The model under review builds one solid part; all positions refer to its coordinate system, in mm. A direction names the side the tool comes from. Round coordinates to 2 decimals unless told otherwise and drop trailing zeros. Loops run counter-clockwise (first coordinate to the right, second up) from the corner with the lowest first, then second, coordinate; pieces in that order, holes last. Notation, with made-up numbers: (36, -7) -> (69, -7) arc R28 cw to (69, 11) -> close; hole circle Ø4 at (-24.75, 88). An arc over 180 degrees is marked (long way). Use CSV: the item, a comma, the result in double quotes. Start each with the question number.
```python
from build123d import *

# Parameters (mm, degrees)
F0_R     = 7.366
F0_R_2   = 5.7785
F1_DEPTH = 1
F2_DEPTH = 2.032
F4_DEPTH = 7.366


with BuildPart() as f1:
    # F0 (on Top) → F1 (new body)
    with BuildSketch(Plane.XY):
        Circle(F0_R)
        Circle(F0_R_2, mode=Mode.SUBTRACT)
        Circle(F0_R_2)
    extrude(amount=F1_DEPTH)

    # F0 (on Top) → F2 (join)
    with BuildSketch(Plane.XY):
        Circle(F0_R)
        Circle(F0_R_2, mode=Mode.SUBTRACT)
    extrude(amount=F2_DEPTH)

    # F3 (on face) → F4 (join)
    with BuildSketch(Plane.XY.offset(1)):
        with BuildLine():
            ThreePointArc((-3.1130078892, 3.687744281), (0, 4.826), (3.1130078892, 3.687744281))
            Line((3.1130078892, 3.687744281), (3.7885305572, 4.3632669489))
            ThreePointArc((3.7885305572, 4.3632669489), (0, 5.7785), (-3.7885305572, 4.3632669489))
            Line((-3.7885305572, 4.3632669489), (-3.1130078892, 3.687744281))
        make_face()
        with BuildLine():
            ThreePointArc((-3.687744281, -3.1130078892), (-4.826, 0), (-3.687744281, 3.1130078892))
            Line((-3.687744281, 3.1130078892), (-4.3632669489, 3.7885305572))
            ThreePointArc((-4.3632669489, 3.7885305572), (-5.7785, 0), (-4.3632669489, -3.7885305572))
            Line((-4.3632669489, -3.7885305572), (-3.687744281, -3.1130078892))
        make_face()
        with BuildLine():
            Line((3.7885305572, -4.3632669489), (3.1130078892, -3.687744281))
            ThreePointArc((3.1130078892, -3.687744281), (0, -4.826), (-3.1130078892, -3.687744281))
            Line((-3.1130078892, -3.687744281), (-3.7885305572, -4.3632669489))
            ThreePointArc((-3.7885305572, -4.3632669489), (0, -5.7785), (3.7885305572, -4.3632669489))
        make_face()
        with BuildLine():
            ThreePointArc((3.687744281, 3.1130078892), (4.5325119912, 1.6572902733), (4.826, 0))
            ThreePointArc((4.826, 0), (4.5325119912, -1.6572902733), (3.687744281, -3.1130078892))
            Line((3.687744281, -3.1130078892), (4.3632669489, -3.7885305572))
            ThreePointArc((4.3632669489, -3.7885305572), (5.4131414315, -2.0221182193), (5.7785, 0))
            ThreePointArc((5.7785, 0), (5.4131414315, 2.0221182193), (4.3632669489, 3.7885305572))
            Line((4.3632669489, 3.7885305572), (3.687744281, 3.1130078892))
        make_face()
    extrude(amount=F4_DEPTH)


solid = f1.part
```
1. For line 1 along Z through (x, y) = (2.75, -0.5); line 2 along Y through (x, z) = (-0.25, 3.75); line 3 along Y through (x, z) = (-2.5, 3.5), list the stretches that pass through material, from the lowest coordinate up. Write a range as from..to.
2. Take a section at C-C, the plane x = 0. Give the boundary of the cut face in (y, z).
3. Take a section at B-B, the plane z = 1.75. Give the boundary of the cut face in (x, y), then the cut area to 3 significant figures.
4. For faces 1 (the face through (0, 0, 1)), 2 (the face through (-5.78, 0.06, 5.15)), 3 (the face through (0.06, 5.78, 5.15)), list the 3-axis set-ups (+Z, -Z, +X, -X, +Y, -Y) from which the entire face can be reached by the end or side of a thin tool; tool diameter is ignored.
5. Clearance check with a flat-ended pin moving along its axis: P1, Ø2, axis at y = -2, z = 2, coming from the +X side. State where the tip first meets the part, or that it passes through.
6. Take a section at A-A, the plane z = 7. Give the boundary of the cut face in (x, y), then the cut area to 3 significant figures.
7. The part is to be moulded in two halves that separate along X. For faces 4 (the face through (0.047, -4.826, 4.631)), 5 (the face through (-4.826, -0.047, 4.631)), 6 (the face through (5, 0, 8.366)), 7 (the face through (-0.06, -5.78, 5.15)), say which applies: pulls with the +X half, pulls with the -X half, needs draft (parallel to the pull), parting line crosses it, or undercut.
8. Take a section at D-D, the plane y = -1.5. Give the boundary of the cut face in (x, z).
Results:
1,line 1,"0..1"
1,line 2,"-5.77..-4.82, 4.82..5.77"
1,line 3,"-5.21..-4.13, 4.13..5.21"
2,outline,"(-7.37, 0) -> (7.37, 0) -> (7.37, 2.03) -> (5.78, 2.03) -> (5.78, 8.37) -> (4.83, 8.37) -> (4.83, 1) -> (-4.83, 1) -> (-4.83, 8.37) -> (-5.78, 8.37) -> (-5.78, 2.03) -> (-7.37, 2.03) -> close"
3,outline,"circle Ø14.73 at (0, 0); hole (-4.36, -3.79) arc R5.78 ccw to (-3.79, -4.36) -> (-3.11, -3.69) arc R4.83 ccw to (3.11, -3.69) -> (3.79, -4.36) arc R5.78 ccw to (4.36, -3.79) -> (3.69, -3.11) arc R4.83 ccw to (3.69, 3.11) -> (4.36, 3.79) arc R5.78 ccw to (3.79, 4.36) -> (3.11, 3.69) arc R4.83 ccw to (-3.11, 3.69) -> (-3.79, 4.36) arc R5.78 ccw to (-4.36, 3.79) -> (-3.69, 3.11) arc R4.83 ccw to (-3.69, -3.11) -> close"
3,area,"94.2 mm²"
4,face 1,"+Z"
4,face 2,"+Z, -X"
4,face 3,"+Z, +Y"
5,P1,"x = 7.3"
6,outline,"(-4.36, -3.79) -> (-3.69, -3.11) arc R4.83 cw to (-3.69, 3.11) -> (-4.36, 3.79) arc R5.78 ccw to start; (-3.79, -4.36) arc R5.78 ccw to (3.79, -4.36) -> (3.11, -3.69) arc R4.83 cw to (-3.11, -3.69) -> close; (-3.79, 4.36) -> (-3.11, 3.69) arc R4.83 cw to (3.11, 3.69) -> (3.79, 4.36) arc R5.78 ccw to start; (3.69, -3.11) -> (4.36, -3.79) arc R5.78 ccw to (4.36, 3.79) -> (3.69, 3.11) arc R4.83 cw to start"
6,area,"28.6 mm²"
7,face 4,"undercut"
7,face 5,"undercut"
7,face 6,"needs draft"
7,face 7,"parting line crosses it"
8,outline,"(-7.21, 0) -> (7.21, 0) -> (7.21, 2.03) -> (5.58, 2.03) -> (5.58, 8.37) -> (4.59, 8.37) -> (4.59, 1) -> (-4.59, 1) -> (-4.59, 8.37) -> (-5.58, 8.37) -> (-5.58, 2.03) -> (-7.21, 2.03) -> close"
